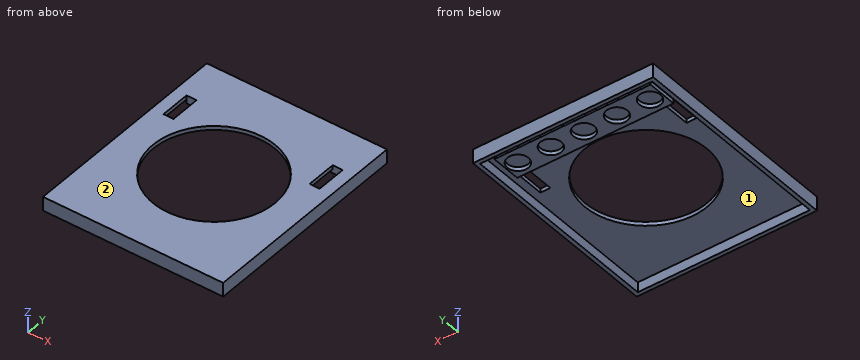
from build123d import *

# Parameters (mm, degrees)
SKETCH043_W         = 90
SKETCH043_H         = 106.9
PAD015_DEPTH        = 7
SKETCH044_W         = 86
SKETCH044_H         = 102.9
POCKET025_DEPTH     = 5
SKETCH045_R         = 30.5
POCKET026_DEPTH     = 2
SKETCH060_W         = 78
SKETCH060_H         = 15
PAD019_DEPTH        = 2
SKETCH061_R         = 5.25
POCKET038_DEPTH     = 2
LINEARPATTERN_COUNT = 5
LINEARPATTERN_PITCH = 16.5
SKETCH062_W         = 5
SKETCH062_H         = 15
POCKET039_DEPTH     = 7.001


with BuildPart() as part:
    # Sketch043 → Pad015 (new body)
    with BuildSketch(Plane.XY):
        with Locations((0, -10.35)):
            Rectangle(SKETCH043_W, SKETCH043_H)
    extrude(amount=PAD015_DEPTH)

    # Sketch044 (on Face5 of Pad015) → Pocket025 (cut)
    with BuildSketch(Plane(origin=(0, 0, 0), x_dir=(1, 0, 0), z_dir=(0, 0, -1))):
        with Locations((0, 10.35)):
            Rectangle(SKETCH044_W, SKETCH044_H)
    extrude(amount=-POCKET025_DEPTH, mode=Mode.SUBTRACT)

    # Sketch045 (on Face5 of Pocket025) → Pocket026 (cut)
    with BuildSketch(Plane.XY.offset(7)):
        with Locations((0, -11)):
            Circle(SKETCH045_R)
    extrude(amount=-POCKET026_DEPTH, mode=Mode.SUBTRACT)

    # Sketch060 (on Face12 of Pocket026) → Pad019 (join)
    with BuildSketch(Plane(origin=(0, 0, 5), x_dir=(1, 0, 0), z_dir=(0, 0, -1))):
        with Locations((0, -29.5)):
            Rectangle(SKETCH060_W, SKETCH060_H)
    extrude(amount=PAD019_DEPTH)

    # Sketch061 (on Face17 of Pad019) → Pocket038 (cut)
    with BuildSketch(Plane(origin=(0, 0, 3), x_dir=(1, 0, 0), z_dir=(0, 0, -1))):
        with Locations((-33, -29.5)):
            Circle(SKETCH061_R)
    pocket038 = extrude(amount=-POCKET038_DEPTH, mode=Mode.SUBTRACT)

    # LinearPattern: Pocket038 ×5
    with Locations(*[(i * LINEARPATTERN_PITCH, 0, 0) for i in range(1, LINEARPATTERN_COUNT)]):
        add(pocket038, mode=Mode.SUBTRACT)

    # Sketch062 (on Face5 of LinearPattern) → Pocket039 (cut, through all)
    with BuildSketch(Plane.XY.offset(7)):
        with Locations((-36.5, 14.5)):
            Rectangle(SKETCH062_W, SKETCH062_H)
        with Locations((36.5, 14.5)):
            Rectangle(SKETCH062_W, SKETCH062_H)
    extrude(amount=-POCKET039_DEPTH, mode=Mode.SUBTRACT)


with BuildPart() as part_1:
    # Body002 placement: moved
    add(part.part.moved(Location((0, 0, 25))))


solid = part_1.part
The listing builds one solid part. Answer for the finished solid, in the listing's coordinates (mm). Face numbers are marked on the shaded views. Give positions to 0.01 mm unless a question says otherwise; leave off trailing zeros. Loops run counter-clockwise (first coordinate to the right, second up) from the corner with the lowest first, then second, coordinate; pieces in that order, holes last. Notation, with made-up numbers: M 2.5,77 L 48.5,77 A27 ccw 48.5,104 Z; hole C 77.25,3.5 d2. An arc over 180 degrees is marked long. Answer as CSV lines item,"result".
Item 1: The part is cut by section C-C (y = -32). Give the vertices of the cut face in (x, z).
Values follow:
outline,"M -45,25 L -43,25 L -43,30 L -22.12,30 L -22.12,32 L -45,32 Z; M 22.12,30 L 43,30 L 43,25 L 45,25 L 45,32 L 22.12,32 Z"
Item 2: Given pin 1 Ø6.5 at (x, y) = (-33, 29.5) entering from -Z; pin 2 Ø11.5 at (x, y) = (-14, 30) entering from -Z, each flat-ended and moving along its own axis, determine where each tip first touches the part or whether it passes through.
Values follow:
pin 1,"stops at z = 30"
pin 2,"stops at z = 28"
Item 3: The mould has two halves that part along Y. Classify the marked faces 1 and 2: released by +Y, released by -Y, zero draft, split by the parting line, or undercut.
Values follow:
face 1,"undercut"
face 2,"zero draft"
Item 4: The part is cut by section A-A (x = 0). Give the vertices of the cut face in (y, z), and give its area (3 significant figures).
Values follow:
outline,"M -63.8,25 L -61.8,25 L -61.8,30 L -41.5,30 L -41.5,32 L -63.8,32 Z; M 19.5,30 L 22,30 L 22,28 L 24.25,28 L 24.25,30 L 34.75,30 L 34.75,28 L 37,28 L 37,30 L 41.1,30 L 41.1,25 L 43.1,25 L 43.1,32 L 19.5,32 Z"
area,"121 mm^2"
Item 5: Straight lines are drawn through the part: line 1 along Y through (x, z) = (-9, 29.75); line 2 along Y through (x, z) = (33, 29.55); line 3 along X through (y, z) = (-21.5, 25.5). For each, find the intervals that lie inside material, in ascending order. Write a range as [from, to].
Values follow:
line 1,"y = [-63.8, -61.8], [22, 37], [41.1, 43.1]"
line 2,"y = [-63.8, -61.8], [22, 24.25], [34.75, 37], [41.1, 43.1]"
line 3,"x = [-45, -43], [43, 45]"
Item 6: The part is cut by section D-D (x = 24.5). Give the vertices of the cut face in (y, z), and give its area (3 significant figures).
Values follow:
outline,"M -63.8,25 L -61.8,25 L -61.8,30 L -29.17,30 L -29.17,32 L -63.8,32 Z; M 7.17,30 L 22,30 L 22,28 L 37,28 L 37,30 L 41.1,30 L 41.1,25 L 43.1,25 L 43.1,32 L 7.17,32 Z"
area,"191 mm^2"
